```python
from build123d import *

# Parameters (mm, degrees)
CROQUIS2_R              = 1.5
CROQUIS2_R_2            = 0.5
SALIENTE_EXTRUIR1_DEPTH = 3


with BuildPart() as part:
    # Croquis2 → Saliente-Extruir1 (new body)
    with BuildSketch(Plane.XY):
        with BuildLine():
            Line((-1, 40), (0, 40))
            ThreePointArc((0, 40), (2.237600264, 36.385035848), (-1.995875264, 35.994516047))
            ThreePointArc((-1.995875264, 35.994516047), (-5.603547267, 37.933990418), (-9.423373519, 36.455550183))
            ThreePointArc((-9.423373519, 36.455550183), (-11.063498127, 36.109866963), (-12, 37.5))
            ThreePointArc((-12, 37.5), (-10.872626967, 43.792559296), (-7.630752828, 49.302325581))
            ThreePointArc((-7.630752828, 49.302325581), (-6.948145724, 49.817230195), (-6.112876654, 50))
            Line((-6.112876654, 50), (-5, 50))
            ThreePointArc((-5, 50), (-5.747548784, 47.549509757), (-6, 45))
            ThreePointArc((-6, 45), (-4.535533906, 41.464466094), (-1, 40))
        make_face()
        with Locations((0, 37.5)):
            Circle(CROQUIS2_R, mode=Mode.SUBTRACT)
        with Locations((-10.5, 37.5)):
            Circle(CROQUIS2_R_2, mode=Mode.SUBTRACT)
    extrude(amount=SALIENTE_EXTRUIR1_DEPTH)


solid = part.part
```
Design review of the part built by this model. Coordinates are the model's own, in mm. A direction names the side the tool comes from. Coordinates: 2 decimals unless noted, no trailing zeros. Loops run counter-clockwise (first coordinate to the right, second up) from the corner with the lowest first, then second, coordinate; pieces in that order, holes last.
Q1. Tool access review of faces 1 (the face through (-5.74, 47.58, 1.48)), 2 (the face through (2, 36, 1)): name each direction out of +Z, -Z, +X, -X, +Y, -Y from which nothing blocks a thin tool from reaching the whole face with its end or side.
Reported:
face 1: +Z, -Z, +X
face 2: +Z, -Z
Q2. The part is to be moulded in two halves that separate along Y. For faces 3 (the face through (-5.54, 37.93, 1.48)), 4 (the face through (-5, 42, 1)), 5 (the face through (-0.5, 40, 1.5)), say which applies: +Y half, -Y half, draft (parallel to the pull), parting line (faces both ways), or undercut.
Reported:
face 3: -Y half
face 4: undercut
face 5: +Y half
Q3. We need section C-C on y = 39.5. State the section outline as (x, z) points, and give its area (3 significant figures).
Reported:
outline: (-11.89, 0) - (1.5, 0) - (1.5, 3) - (-11.89, 3) - close
area: 40.2 mm2
Q4. We need section A-A on x = -10.5. State the section outline as (y, z) points.
Reported:
outline: (36, 0) - (37, 0) - (37, 3) - (36, 3) - close; (38, 0) - (44.72, 0) - (44.72, 3) - (38, 3) - close
Q5. We need section B-B on z = 1.15. State the section outline as (x, y) points (3 decimals), and give its area (3 significant figures).
Reported:
outline: (-12, 37.5) arc R1.5 ccw to (-9.423, 36.456) arc R4.899 cw to (-1.996, 35.995) arc R2.5 ccw (long way) to (0, 40) - (-1, 40) arc R5 cw to (-6, 45) arc R13 cw to (-5, 50) - (-6.113, 50) arc R2 ccw to (-7.631, 49.302) arc R18.125 ccw to start; hole circle Ø1 at (-10.5, 37.5); hole circle Ø3 at (0, 37.5)
area: 87.6 mm2
Q6. For pin 1 (1.5 mm diameter, centred on x = -1, z = 1.5, fed in from -Y); pin 2 (4 mm diameter, centred on x = -9.5, y = 40.5, fed in from -Z); pin 3 (1.5 mm diameter, centred on y = 38.5, z = 2.5, fed in from -X); pin 4 (1 mm diameter, centred on x = -7, z = 0.5, fed in from +Y), all flat-tipped, find the tip position at first contact; note any pin that passes through.
Reported:
pin 1: stops at y = 35.01
pin 2: stops at z = 0
pin 3: stops at x = -12
pin 4: stops at y = 49.96
Q7. We need section D-D on x = -2.5. State the section outline as (y, z) points, and give its area (3 significant figures).
Reported:
outline: (36.56, 0) - (40.23, 0) - (40.23, 3) - (36.56, 3) - close
area: 11.0 mm2
Q8. To check wall thickness, follow line 1 (Y direction, x = 0, z = 0.7); line 2 (Y direction, x = -10.5, z = 0.75); line 3 (Y direction, x = -6.5, z = 0.7). State the ranges of each line that lie inside material, in increasing order.
Reported:
line 1: y = 35 to 36, 39 to 40
line 2: y = 36 to 37, 38 to 44.72
line 3: y = 37.91 to 49.96
